from build123d import *

# Parameters (mm, degrees)
F0_W     = 147.200812
F0_H     = 99.25572
F1_DEPTH = 75.438
F4_DEPTH = 44.704
F6_DEPTH = 65.278


with BuildPart() as f1:
    # F0 (on Front) → F1 (new body)
    with BuildSketch(Plane.XZ):
        with Locations((13.084514, -25.390397)):
            Rectangle(F0_W, F0_H)
    extrude(amount=F1_DEPTH)

    # F2 (on face) → F4 (cut)
    with BuildSketch(Plane.XY.offset(24.237463)):
        Polygon((86.68492, -75.438), (86.68492, 0), (31.858269, -75.438), align=None)
    extrude(amount=-F4_DEPTH, mode=Mode.SUBTRACT)

    # F5 (on face) → F6 (join)
    with BuildSketch(Plane.YZ.offset(86.68492)):
        Polygon((-46.992108, -2.242462), (-75.438, -18.509679), (-75.438, -23.966648), (0, -23.966648), (0, 24.237463), align=None)
    extrude(amount=-F6_DEPTH)


solid = f1.part
The listing builds one solid part. Answer for the finished solid, in the listing's coordinates (mm). A direction names the side the tool comes from. Round coordinates to 2 decimals unless told otherwise and drop trailing zeros. Order: outer loops, then holes, each group sorted by start corner. A loop starts at its lowest first (then second) coordinate and runs counter-clockwise, first axis right, second up. Notation, with made-up numbers: (9, 43.25) -> (25, 43.25) arc R33 ccw to (25, 73.25) -> close; hole circle Ø7 at (40.5, 12). An arc over 180 degrees is marked (long way). One line per item, written item: value.
Item 1: Find section B-B, the plane y = -61. Give the vertices of the cut face in (x, z).
Taken from the geometry:
outline: (-60.52, -75.02) -> (86.68, -75.02) -> (86.68, -10.25) -> (42.35, -10.25) -> (42.35, 24.24) -> (-60.52, 24.24) -> close
Item 2: For faces 1 (the flat face through (12, -37, -75.018)), 2 (the flat face through (77.44, -33.61, 5.3)), determine the directions among +Z, -Z, +X, -X, +Y, -Y from which every point of the face is accessible in a straight line to the end or side of a thin tool.
Taken from the geometry:
face 1: -Z, +X, -X, +Y, -Y
face 2: +Z, +X, -Y
Item 3: Straight lines are drawn through the part: L1, parallel to X at y = -54, z = 4.5; L2, parallel to X at y = -58.5, z = -3.5; L3, parallel to Z at x = 79, y = -36. For each, find the intervals that lie inside material, in ascending order.
Taken from the geometry:
L1: x = -60.52 to 47.44
L2: x = -60.52 to 44.17
L3: z = -75.02 to 3.95
Item 4: Find section A-A, the plane x = 76.5. Give the vertices of the cut face in (y, z), then the cut area to 3 significant figures.
Taken from the geometry:
outline: (-75.44, -75.02) -> (0, -75.02) -> (0, 24.24) -> (-14.01, 24.24) -> (-14.01, 16.34) -> (-46.99, -2.24) -> (-75.44, -18.51) -> close
area: 5,940 mm2
Item 5: Find section C-C, the plane z = 0.5. Give the vertices of the cut face in (x, y), then the cut area to 3 significant figures.
Taken from the geometry:
outline: (-60.52, -75.44) -> (31.86, -75.44) -> (56.07, -42.13) -> (86.68, -42.13) -> (86.68, 0) -> (-60.52, 0) -> close
area: 9,680 mm2
